from build123d import *

# Parameters (mm, degrees)
SKETCH1_W           = 100
SKETCH1_H           = 40
BOSS_EXTRUDE1_DEPTH = 10
SKETCH2_R           = 4
BOSS_EXTRUDE2_DEPTH = 10


with BuildPart() as part:
    # Sketch1 → Boss-Extrude1 (new body)
    with BuildSketch(Plane(origin=(0, 0, 0), x_dir=(0, 0, -1), z_dir=(1, 0, 0))):
        Rectangle(SKETCH1_W, SKETCH1_H)
    extrude(amount=BOSS_EXTRUDE1_DEPTH)

    # Sketch2 → Boss-Extrude2 (add)
    with BuildSketch(Plane(origin=(10, 0, 0), x_dir=(0, 0, -1), z_dir=(1, 0, 0))):
        with Locations((18, -5)):
            Circle(SKETCH2_R)
        with Locations((8, -5)):
            Circle(SKETCH2_R)
        with Locations((-2, -5)):
            Circle(SKETCH2_R)
        with Locations((-12, -5)):
            Circle(SKETCH2_R)
    extrude(amount=BOSS_EXTRUDE2_DEPTH)


solid = part.part
CAD build for the part. Positions are in the model's coordinates, mm. A direction names the side the tool comes from. Round coordinates to 2 decimals unless told otherwise and drop trailing zeros. Write each loop counter-clockwise with the first axis right and the second up, starting at its lowest first coordinate (ties: lowest second). Pieces come first, ordered by that corner, then holes. Notation, with made-up numbers: (42, 20.5) -> (55, 20.5) arc R24 ccw to (55, 49.5) -> close; hole circle Ø8 at (-40, 15). An arc over 180 degrees is marked (long way). Answer as a JSON object with one key per item and string values.
(1) Band-saw the part on C-C, the plane y = -17. List the corners of the cut face in (x, z), then the cut area to 3 significant figures.
Reported:
{"outline": "(0, -50) -> (10, -50) -> (10, 50) -> (0, 50) -> close", "area": "1,000 mm^2"}
(2) Band-saw the part on B-B, the plane z = 12. List the corners of the cut face in (x, y).
Reported:
{"outline": "(0, -20) -> (10, -20) -> (10, -9) -> (20, -9) -> (20, -1) -> (10, -1) -> (10, 20) -> (0, 20) -> close"}
(3) Which spindle directions (+Z, -Z, +X, -X, +Y, -Y) get a long thin tool onto all of the face, cutting with end or side? Do faces 1 (the face through (14.9, -7.4, 15.2)), 2 (the face through (5, 20, 1)). Say none if no direction does.
Reported:
{"face 1": "+X", "face 2": "+Z, -Z, +X, -X, +Y"}
(4) Two-plate mould, pull along Z, no slides. Class faces 3 (the face through (5, 0, -50)), 4 (the face through (5, 0, 50)), 5 (the face through (14.9, -7.4, -4.8)), 6 (the face through (20, -5, 12)): +Z half, -Z half, draft (parallel to the pull), parting line (faces both ways), or undercut.
Reported:
{"face 3": "-Z half", "face 4": "+Z half", "face 5": "undercut", "face 6": "draft"}
(5) Probe probe 1 along Z at (x, y) = (12.5, -4.5); probe 2 along Z at (x, y) = (10.75, -4); probe 3 along X at (y, z) = (10, 9). List the from-to ranges inside material, lowest first. Write a range as [from, to].
Reported:
{"probe 1": "z = [-21.97, -14.03], [-11.97, -4.03], [-1.97, 5.97], [8.03, 15.97]", "probe 2": "z = [-21.87, -14.13], [-11.87, -4.13], [-1.87, 5.87], [8.13, 15.87]", "probe 3": "x = [0, 10]"}
(6) Band-saw the part on A-A, the plane x = 17.25. List the corners of the cut face in (y, z), then the cut area to 3 significant figures.
Reported:
{"outline": "circle Ø8 at (-5, -18); circle Ø8 at (-5, -8); circle Ø8 at (-5, 2); circle Ø8 at (-5, 12)", "area": "201 mm^2"}
(7) Pin check, flat tips, straight feed: P1, Ø3, axis at x = 12, z = -9.5, coming from the -Y side; P2, Ø10, axis at x = 17, y = -12.5, coming from the -Z side; P3, Ø4, axis at x = 16.5, y = -10.5, coming from the +Z side. Stop position of each tip, or through.
Reported:
{"P1": "stops at y = -9", "P2": "stops at z = -21.12", "P3": "stops at z = 13.94"}
